```python
from build123d import *

# Parameters (mm, degrees)
F0_R     = 1.524
F1_DEPTH = 5.08
F2_ANGLE = 180
F3_ANGLE = 180
F4_R     = 3.175
F4_R_2   = 1.524
F5_DEPTH = 2.54
F6_R     = 5.08


with BuildPart() as f1:
    # F0 (on Top) → F1 (new body)
    with BuildSketch(Plane.XY):
        Polygon((0, 15.24), (0, 0), (71.12, 0), (71.12, 15.24), (53.0225, 15.24), (52.07, 15.24), (20.0025, 15.24), (19.05, 15.24), align=None)
        with Locations((7.62, 6.35)):
            Circle(F0_R, mode=Mode.SUBTRACT)
        with Locations((63.5, 6.35)):
            Circle(F0_R, mode=Mode.SUBTRACT)
    extrude(amount=F1_DEPTH)

    # F0 (on Top) → F2 (revolve)
    with BuildSketch(Plane.XY):
        Polygon((19.05, 18.796), (19.05, 15.24), (20.0025, 15.24), (20.0025, 17.78), (22.352, 17.78), (22.352, 18.796), align=None)
    revolve(axis=Axis((19.05, 5.626085, 0), (0, -1, 0)), revolution_arc=F2_ANGLE)

    # F0 (on Top) → F3 (revolve)
    with BuildSketch(Plane.XY):
        Polygon((52.07, 15.24), (53.0225, 15.24), (53.0225, 17.78), (55.372, 17.78), (55.372, 18.796), (52.07, 18.796), align=None)
    revolve(axis=Axis((52.07, 5.626085, 0), (0, -1, 0)), revolution_arc=F3_ANGLE)

    # F4 (on face) → F5 (cut)
    with BuildSketch(Plane.XY.offset(5.08)):
        with Locations((7.62, 6.35)):
            Circle(F4_R)
        with Locations((7.62, 6.35)):
            Circle(F4_R_2, mode=Mode.SUBTRACT)
        with Locations((63.5, 6.35)):
            Circle(F4_R)
        with Locations((63.5, 6.35)):
            Circle(F4_R_2, mode=Mode.SUBTRACT)
    extrude(amount=-F5_DEPTH, mode=Mode.SUBTRACT)

    # F6
    f6_edges = [f1.edges().sort_by_distance(p)[0] for p in [
        (71.12, 15.24, 2.54),
        (71.12, 0, 2.54),
        (0, 15.24, 2.54),
        (0, 0, 2.54),
    ]]
    fillet(f6_edges, radius=F6_R)


solid = f1.part
```
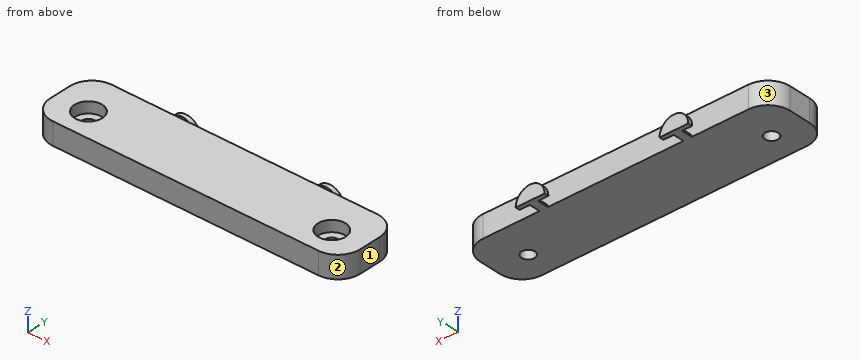
The listing builds one solid part. Answer for the finished solid, in the listing's coordinates (mm). Face numbers are marked on the shaded views. Coordinates: 2 decimals unless noted, no trailing zeros. Loops run counter-clockwise (first coordinate to the right, second up) from the corner with the lowest first, then second, coordinate; pieces in that order, holes last. Notation, with made-up numbers: (46.5, 81.25) -> (81.5, 81.25) arc R32 cw to (81.5, 117.25) -> close; hole circle Ø7 at (43, -15.5). An arc over 180 degrees is marked (long way). Return JSON: item names as keys, results as strings. Group by question number.
(1) A cutting plane is placed at D-D on x = 52.07. Write down the section's boundary in (y, z), and give its area (3 significant figures).
(2) A cutting plane is placed at C-C on z = 1.8. Write down the section's boundary in (x, y).
(3) A cutting plane is placed at B-B on y = 6.35. Write down the section's boundary in (x, z) (3 decimals).
(4) Given pin 1 Ø8.5 at (x, y) = (63.5, 6.35) entering from -Z; pin 2 Ø3 at (y, z) = (13.5, 3.5) entering from +X; pin 3 Ø1.9 at (x, y) = (7, 7) entering from +Z, each flat-ended and moving along its own axis, determine where each tip first touches the part or whether it passes through.
(5) Find the intervals of material crossed by probe 1 along X at (y, z) = (4.5, 4.4); probe 2 along Y at (x, z) = (63.5, 0.7); probe 3 along Y at (x, z) = (63.5, 4.25) (3 decimals), in increasing order. Write a range as from..to.
(6) A cutting plane is placed at A-A on x = 7.62. Write down the section's boundary in (y, z) (3 decimals).
(7) Determine the mould class of the marked faces 1, 2 and 3 for opening direction Y: released by +Y, released by -Y, zero draft, split by the parting line, or undercut.
The answers:
{
 "1": {"outline": "(0, 0) -> (18.8, 0) -> (18.8, 3.3) -> (17.78, 3.3) -> (17.78, 0.95) -> (15.24, 0.95) -> (15.24, 5.08) -> (0, 5.08) -> close", "area": "83.2 mm^2"},
 "2": {"outline": "(0, 5.08) arc R5.08 ccw to (5.08, 0) -> (66.04, 0) arc R5.08 ccw to (71.12, 5.08) -> (71.12, 10.16) arc R5.08 ccw to (66.04, 15.24) -> (5.08, 15.24) arc R5.08 ccw to (0, 10.16) -> close; (16.28, 17.78) -> (21.82, 17.78) -> (21.82, 18.8) -> (16.28, 18.8) -> close; (49.3, 17.78) -> (54.84, 17.78) -> (54.84, 18.8) -> (49.3, 18.8) -> close; hole circle Ø3.05 at (7.62, 6.35); hole circle Ø3.05 at (63.5, 6.35)"},
 "3": {"outline": "(0, 0) -> (6.096, 0) -> (6.096, 2.54) -> (4.445, 2.54) -> (4.445, 5.08) -> (0, 5.08) -> close; (9.144, 0) -> (61.976, 0) -> (61.976, 2.54) -> (60.325, 2.54) -> (60.325, 5.08) -> (10.795, 5.08) -> (10.795, 2.54) -> (9.144, 2.54) -> close; (65.024, 0) -> (71.12, 0) -> (71.12, 5.08) -> (66.675, 5.08) -> (66.675, 2.54) -> (65.024, 2.54) -> close"},
 "4": {"pin 1": "stops at z = 0", "pin 2": "stops at x = 70.78", "pin 3": "stops at z = 2.54"},
 "5": {"probe 1": "x = 0.03..5.04, 10.2..60.92, 66.08..71.09", "probe 2": "y = 0..4.83, 7.87..15.24", "probe 3": "y = 0..3.175, 9.525..15.24"},
 "6": {"outline": "(0, 0) -> (4.826, 0) -> (4.826, 2.54) -> (3.175, 2.54) -> (3.175, 5.08) -> (0, 5.08) -> close; (7.874, 0) -> (15.24, 0) -> (15.24, 5.08) -> (9.525, 5.08) -> (9.525, 2.54) -> (7.874, 2.54) -> close"},
 "7": {"face 1": "zero draft", "face 2": "released by -Y", "face 3": "released by +Y"}
}
